Geometry check sheet. Reference: the model listing, model coordinates, mm. Face numbers are marked on the shaded views. A direction names the side the tool comes from. Give positions to 0.01 mm unless a question says otherwise; leave off trailing zeros. Loops run counter-clockwise (first coordinate to the right, second up) from the corner with the lowest first, then second, coordinate; pieces in that order, holes last.
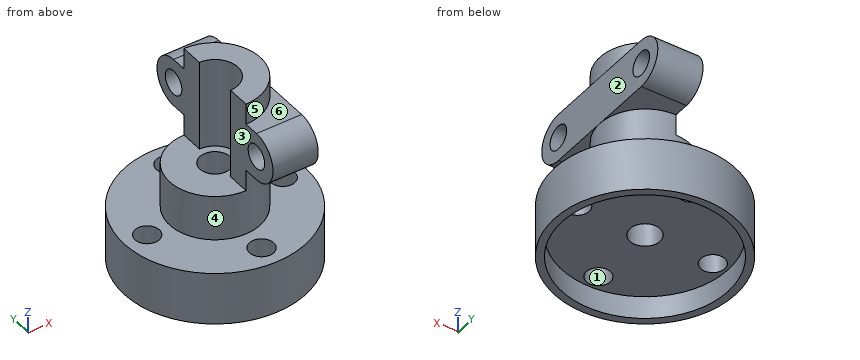
```python
from build123d import *

# Parameters (mm, degrees)
SKETCH1_R               = 60
SKETCH1_R_2             = 30
BOSS_EXTRUDE1_DEPTH     = 35
SKETCH1_3_R             = 30
BOSS_EXTRUDE2_DEPTH     = 125
BOSS_EXTRUDE3_DEPTH     = 30
CUT_EXTRUDE2_DEPTH      = 152.079449297
CUT_EXTRUDE2_DEPTH_BACK = 152.079449297
SKETCH5_R               = 10
CUT_EXTRUDE3_DEPTH      = 152.079449297
CUT_EXTRUDE3_DEPTH_BACK = 60
CUT_EXTRUDE4_DEPTH      = 60
SKETCH9_R               = 8
CUT_EXTRUDE5_DEPTH      = 166.302752548
SKETCH10_R              = 8
CUT_EXTRUDE6_DEPTH      = 124.693168769
SKETCH11_R              = 55
CUT_EXTRUDE7_DEPTH      = 15


with BuildPart() as part:
    # Sketch1 → Boss-Extrude1 (new body)
    # profile 1 of 2: a face of its own
    with BuildSketch(Plane(origin=(0, 0, 0), x_dir=(0, 1, 0), z_dir=(0, 0, 1))):
        with Locations(Location((0, 0, 0), (0, 0, 270))):
            Circle(SKETCH1_R)
        Circle(SKETCH1_R_2, mode=Mode.SUBTRACT)
    # profile 2 of 2: a face of its own
    with BuildSketch(Plane(origin=(0, 0, 0), x_dir=(0, 1, 0), z_dir=(0, 0, 1))):
        Circle(SKETCH1_R_2)
    extrude(amount=BOSS_EXTRUDE1_DEPTH)

    # Sketch1<3> → Boss-Extrude2 (add)
    with BuildSketch(Plane(origin=(0, 0, 0), x_dir=(0, 1, 0), z_dir=(0, 0, 1))):
        with Locations(Location((0, 0, 0), (0, 0, 270))):
            Circle(SKETCH1_3_R)
    extrude(amount=BOSS_EXTRUDE2_DEPTH)

    # Sketch4 → Boss-Extrude3 (add)
    with BuildSketch(Plane.YZ):
        with BuildLine():
            Line((40, 79), (-40, 79))
            ThreePointArc((-40, 79), (-56, 95), (-40, 111))
            Line((-40, 111), (40, 111))
            ThreePointArc((40, 111), (56, 95), (40, 79))
        make_face()
    extrude(amount=BOSS_EXTRUDE3_DEPTH)

    # Sketch5 → Cut-Extrude2 (cut, two sides: drawn at the far end of the back side and taken through both)
    with BuildSketch(Plane.XY.offset(125).offset(-CUT_EXTRUDE2_DEPTH_BACK)):
        Circle(SKETCH5_R)
    extrude(amount=CUT_EXTRUDE2_DEPTH + CUT_EXTRUDE2_DEPTH_BACK, mode=Mode.SUBTRACT)

    # Sketch7 → Cut-Extrude3 (cut, two sides: drawn at the far end of the back side and taken through both)
    with BuildSketch(Plane.XY.offset(125).offset(-CUT_EXTRUDE3_DEPTH_BACK)):
        with BuildLine():
            Line((0, 30), (0, -30))
            ThreePointArc((0, -30), (-30, 0), (0, 30))
        make_face()
    extrude(amount=CUT_EXTRUDE3_DEPTH + CUT_EXTRUDE3_DEPTH_BACK, mode=Mode.SUBTRACT)

    # Sketch8 → Cut-Extrude4 (cut)
    with BuildSketch(Plane.XY.offset(125)):
        with BuildLine():
            Line((0, 15), (0, 10))
            ThreePointArc((0, 10), (10, 0), (0, -10))
            Line((0, -10), (0, -15))
            ThreePointArc((0, -15), (15, 0), (0, 15))
        make_face()
    extrude(amount=-CUT_EXTRUDE4_DEPTH, mode=Mode.SUBTRACT)

    # Sketch9 → Cut-Extrude5 (cut, through all)
    with BuildSketch(Plane.YZ.offset(30)):
        with Locations(Location((-40, 95, 0), (0, 0, 270))):
            Circle(SKETCH9_R)
        with Locations(Location((40, 95, 0), (0, 0, 270))):
            Circle(SKETCH9_R)
    extrude(amount=-CUT_EXTRUDE5_DEPTH, mode=Mode.SUBTRACT)

    # Sketch10 → Cut-Extrude6 (cut, through all)
    with BuildSketch(Plane.XY.offset(35)):
        with Locations((-45, 0)):
            Circle(SKETCH10_R)
        with Locations((0, 45)):
            Circle(SKETCH10_R)
        with Locations((45, 0)):
            Circle(SKETCH10_R)
        with Locations((0, -45)):
            Circle(SKETCH10_R)
    extrude(amount=-CUT_EXTRUDE6_DEPTH, mode=Mode.SUBTRACT)

    # Sketch11 → Cut-Extrude7 (cut)
    with BuildSketch(Plane(origin=(0, 0, 0), x_dir=(1, 0, 0), z_dir=(0, 0, -1))):
        with Locations(Location((0, 0, 0), (0, 0, 180))):
            Circle(SKETCH11_R)
    extrude(amount=-CUT_EXTRUDE7_DEPTH, mode=Mode.SUBTRACT)


solid = part.part
```
1) Mould release check, pull along X, two halves, no side actions. Record for the marked faces 1, 2 and 3: +X half, -X half, draft (parallel to the pull), parting line (faces both ways), or undercut.
2) Sectioned sample at D-D on x = 21. Enter the section's corners in (y, z), plus the area to 3 significant figures.
3) Tool access check on the marked faces 4, 5 and 6. Record the directions out of +Z, -Z, +X, -X, +Y, -Y that give a thin tool (end or side, any length) a straight path to the whole face; none if there is none.
4) Sectioned sample at B-B on x = 43.5. Enter the section's corners in (y, z).
5) Depth check by flat-ended pin: P1, Ø5, axis at y = -30.5, z = 34.5, coming from the -X side; P2, Ø15, axis at x = 13, y = 12, coming from the -Z side; P3, Ø13, axis at x = 0, y = 45, coming from the +Z side. Enter the tip coordinate at first touch or a pass-through.
6) Sectioned sample at C-C on z = 94. Enter the section's corners in (x, y), plus the area to 3 significant figures.
7) Sectioned sample at A-A on y = -34. Enter the section's corners in (x, z), plus the area to 3 significant figures.
8) Scan lines: line 1 along Y through (x, z) = (0, 29.75); line 2 along Y through (x, z) = (15.5, 95); line 3 along Z through (x, y) = (22, -30.5). Record each from-to range of solid material in increasing order.
Determined:
1. face 1: undercut
1. face 2: +X half
1. face 3: -X half
2. outline: (-56.2, 0) - (-50.83, 0) - (-50.83, 15) - (50.83, 15) - (50.83, 0) - (56.2, 0) - (56.2, 35) - (21.42, 35) - (21.42, 79) - (40, 79) arc R16 ccw to (40, 111) - (21.42, 111) - (21.42, 125) - (-21.42, 125) - (-21.42, 111) - (-40, 111) arc R16 ccw to (-40, 79) - (-21.42, 79) - (-21.42, 35) - (-56.2, 35) - close; hole circle Ø16 at (-40, 95); hole circle Ø16 at (40, 95)
2. area: 7,860 mm2
3. face 4: none
3. face 5: +Z, +X
3. face 6: +Z, +X, -Y
4. outline: (-41.32, 0) - (-33.66, 0) - (-33.66, 15) - (-7.86, 15) - (-7.86, 35) - (-41.32, 35) - close; (7.86, 15) - (33.66, 15) - (33.66, 0) - (41.32, 0) - (41.32, 35) - (7.86, 35) - close
5. P1: stops at x = -53.07
5. P2: stops at z = 15
5. P3: stops at z = 111
6. outline: (0, -55.97) - (30, -55.97) - (30, -47.94) - (0, -47.94) - close; (0, -32.06) - (30, -32.06) - (30, 32.06) - (0, 32.06) - (0, 15) arc R15 cw to (0, -15) - close; (0, 47.94) - (30, 47.94) - (30, 55.97) - (0, 55.97) - close
6. area: 2,050 mm2
7. outline: (-49.44, 0) - (-43.23, 0) - (-43.23, 15) - (43.23, 15) - (43.23, 0) - (49.44, 0) - (49.44, 35) - (-49.44, 35) - close; (0, 79) - (30, 79) - (30, 89.71) - (0, 89.71) - close; (0, 100.29) - (30, 100.29) - (30, 111) - (0, 111) - close
7. area: 2,810 mm2
8. line 1: y = -60 to -53, -37 to -10, 10 to 37, 53 to 60
8. line 2: y = -56 to -48, -32 to 32, 48 to 56
8. line 3: z = 15 to 35, 79 to 111
